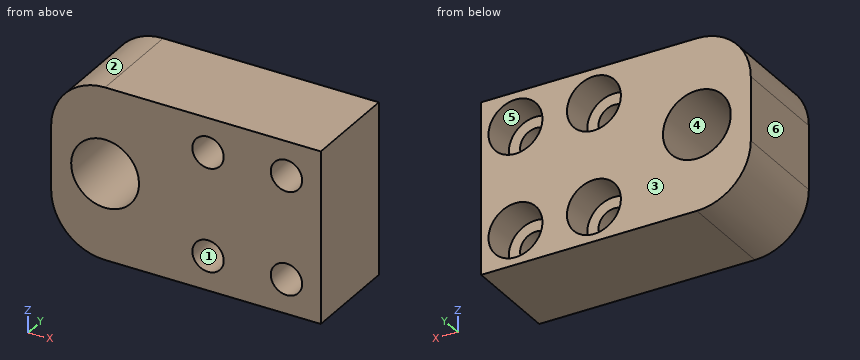
Autodesk Inventor part; units mm, degrees
ref_plane "YZ Plane" through (0, 0, 0) normal (1, 0, 0) x (0, 1, 0)
ref_plane "XZ Plane" through (0, 0, 0) normal (0, 1, 0) x (-1, 0, 0)
ref_plane "XY Plane" through (0, 0, 0) normal (0, 0, 1) x (1, 0, 0)
sketch "Sketch1" plane through (0, 0, 0) normal (0, 1, 0) x (-1, 0, 0)
  line L0 (27.5, 17.5) -> (-27.5, 17.5)
  line L1 (-27.5, 17.5) -> (-27.5, -17.5)
  line L2 (-27.5, -17.5) -> (27.5, -17.5)
  line L3 (27.5, -17.5) -> (27.5, 17.5)
  line L4 (27.5, 17.5) -> (-27.5, -17.5) construction
  line L5 (-27.5, 17.5) -> (27.5, -17.5) construction
  point P0 (0, 0)
  dimension "d0" = 55
  dimension "d1" = 35
extrude "Extrusion1" add sketch "Sketch1" along normal blind 20
sketch "Sketch2" plane through (0, 20, 0) normal (0, 1, 0) x (1, 0, 0)
  circle A0 centre (20.5, 10.5) radius 5.5
  circle A1 centre (20.5, -10.5) radius 5.5
  circle A2 centre (4.5, -10.5) radius 5.5
  circle A3 centre (4.5, 10.5) radius 5.5
  line L0 (27.5, -17.5) -> (27.5, 17.5)
  point P0 (0, 0)
  dimension "d4" = 11
  dimension "d5" = 11
  dimension "d6" = 11
  dimension "d7" = 11
  dimension "d8" = 21
  dimension "d9" = 21
  dimension "d10" = 10.5
  dimension "d11" = 10.5
  dimension "d12" = 23
  dimension "d13" = 23
  dimension "d14" = 7
  dimension "d15" = 7
extrude "Extrusion2" cut sketch "Sketch2" against normal blind 7
sketch "Sketch3" plane through (4.5, 13, 10.5) normal (0, 1, 0) x (1, 0, 0)
  circle A0 centre (0, 0) radius 3.2
  circle A1 centre (0, 21) radius 5.5
  circle A2 centre (16, 21) radius 5.5
  circle A3 centre (16, 0) radius 5.5
  circle A4 centre (0, 21) radius 3.2
  circle A5 centre (16, 21) radius 3.2
  circle A6 centre (16, 0) radius 3.2
  point P0 (-4.5, 10.5)
  dimension "d18" = 6.4
  dimension "d19" = 6.4
  dimension "d20" = 6.4
  dimension "d21" = 6.4
extrude "Extrusion3" cut sketch "Sketch3" against normal blind 20 contours A0 | A4 | A5 | A6
sketch "Sketch4" plane through (0, 20, 0) normal (0, 1, 0) x (1, 0, 0)
  line L0 (27.5, -17.5) -> (27.5, 17.5)
  point P0 (0, 0)
  point P1 (-16.5, 0)
  dimension "d27" = 44
fillet "Fillet1" radius 11 2 edges at (-27.5, 10, 17.5) (-27.5, 10, -17.5)
hole "Hole1" at (-16.5, 20, 0) direction (0, -1, 0) diameter 13.835 depth 41.3 tip angle 118
properties part number "Spindlesocket"
Work out the finished part from the listing and answer in its coordinate system (mm). Face numbers are marked on the shaded views. A direction names the side the tool comes from. Round coordinates to 2 decimals unless told otherwise and drop trailing zeros. Loops run counter-clockwise (first coordinate to the right, second up) from the corner with the lowest first, then second, coordinate; pieces in that order, holes last. Notation, with made-up numbers: M -22,-27.5 L 30,-27.5 A23 cw 30,1.5 Z; hole C -27,10.25 d6. An arc over 180 degrees is marked long. One line per question, with ' | ' between items.
Q1. Find section B-B, the plane x = 20.5. Give the vertices of the cut face in (y, z), then the cut area to 3 significant figures.
Conclusion:
outline: M 0,-17.5 L 20,-17.5 L 20,-16 L 13,-16 L 13,-13.7 L 0,-13.7 Z; M 0,-7.3 L 13,-7.3 L 13,-5 L 20,-5 L 20,5 L 13,5 L 13,7.3 L 0,7.3 Z; M 0,13.7 L 13,13.7 L 13,16 L 20,16 L 20,17.5 L 0,17.5 Z | area: 380 mm2
Q2. Each of these flat-tipped pins is pushed along its axis until it touches: pin 1 Ø10 at (x, z) = (20.5, 10.5) entering from +Y; pin 2 Ø4 at (x, z) = (20.5, -10.5) entering from +Y; pin 3 Ø8 at (y, z) = (14.5, -12) entering from -X. Where does it stop, or does it pass through?
Conclusion:
pin 1: stops at y = 13 | pin 2: passes through | pin 3: stops at x = -27.4
Q3. Consider line 1 along Z through (x, y) = (20.5, 17.75); line 2 along Z through (x, y) = (4.5, 8); line 3 along X through (y, z) = (14.5, -10.5). Determine where each line is inside the solid, lowest interval first. Write a range as from..to.
Conclusion:
line 1: z = -17.5..-16, -5..5, 16..17.5 | line 2: z = -17.5..-13.7, -7.3..7.3, 13.7..17.5 | line 3: x = -26.75..-1, 10..15, 26..27.5
Q4. A tool of negligible diameter and unlimited length cuts with its end or side. For the marked faces 5 and 6, from which of +Z, -Z, +X, -X, +Y, -Y can it reach the whole face along a straight path? Write none if from no direction.
Conclusion:
face 5: +Y | face 6: +Z, -Z, -X, +Y, -Y
Q5. Find section D-D, the plane z = 11.5. Give the vertices of the cut face in (x, y), then the cut area to 3 significant figures.
Conclusion:
outline: M -26.3,0 L 1.46,0 L 1.46,13 L -0.91,13 L -0.91,20 L -26.3,20 Z; M 7.54,0 L 17.46,0 L 17.46,13 L 15.09,13 L 15.09,20 L 9.91,20 L 9.91,13 L 7.54,13 Z; M 23.54,0 L 27.5,0 L 27.5,20 L 25.91,20 L 25.91,13 L 23.54,13 Z | area: 766 mm2
Q6. Find section C-C, the plane z = -1. Give the vertices of the cut face in (x, y).
Conclusion:
outline: M -27.5,0 L -23.34,0 L -23.34,20 L -27.5,20 Z; M -9.66,0 L 27.5,0 L 27.5,20 L -9.66,20 Z
Q7. Find section A-A, the plane y = 11.25. Give the vertices of the cut face in (x, z) (1 decimal), then the cut area to 3 significant figures.
Conclusion:
outline: M -27.5,-6.5 A11 ccw -16.5,-17.5 L 27.5,-17.5 L 27.5,17.5 L -16.5,17.5 A11 ccw -27.5,6.5 Z; hole C -16.5,0 d13.8; hole C 4.5,-10.5 d6.4; hole C 4.5,10.5 d6.4; hole C 20.5,-10.5 d6.4; hole C 20.5,10.5 d6.4 | area: 1,590 mm2
Q8. The mould has two halves that part along Z. Classify the marked faces 1, 2, 3 and 4: +Z half, -Z half, draft (parallel to the pull), parting line (faces both ways), or undercut.
Conclusion:
face 1: undercut | face 2: +Z half | face 3: draft | face 4: undercut
